from build123d import *

# Parameters (mm, degrees)
SKETCH1_W           = 85.2
SKETCH1_H           = 18
SKETCH1_R           = 1.5
BOSS_EXTRUDE1_DEPTH = 18
SKETCH2_R           = 3
CUT_EXTRUDE1_DEPTH  = 8
FILLET1_R           = 4


with BuildPart() as part:
    # Sketch1 → Boss-Extrude1 (new body)
    with BuildSketch(Plane(origin=(0, 0, 0), x_dir=(0, 0, -1), z_dir=(1, 0, 0))):
        with Locations((42.6, 9)):
            Rectangle(SKETCH1_W, SKETCH1_H)
        with Locations((76.2, 9)):
            Circle(SKETCH1_R, mode=Mode.SUBTRACT)
    extrude(amount=BOSS_EXTRUDE1_DEPTH)

    # Sketch2 → Cut-Extrude1 (cut)
    with BuildSketch(Plane.ZY):
        with Locations((-76.2, 9)):
            Circle(SKETCH2_R)
    extrude(amount=-CUT_EXTRUDE1_DEPTH, mode=Mode.SUBTRACT)

    # Fillet1
    fillet1_edges = [part.edges().sort_by_distance(p)[0] for p in [
        (9, 18, -85.2),
        (9, 0, -85.2),
    ]]
    fillet(fillet1_edges, radius=FILLET1_R)


solid = part.part
Input: part model. Units: mm. Frame: model coordinates. A direction names the side the tool comes from. Give positions to 0.01 mm unless a question says otherwise; leave off trailing zeros. Write each loop counter-clockwise with the first axis right and the second up, starting at its lowest first coordinate (ties: lowest second). Pieces come first, ordered by that corner, then holes.
Q1. Section A-A, the plane z = -76.2. Output: boundary loops of the cut face in (x, y), plus the area to 3 significant figures.
Q2. Set-up query: faces 5 (the face through (9.126, 16.859, -83.997)), 6 (the face through (8, 8, -78)). Return all of +Z, -Z, +X, -X, +Y, -Y with unobstructed straight access to the full face (end or side cutting, diameter ignored); none if empty.
Q3. Pull-direction query (Y, two-part tool) for faces 1 (the face through (3.94, 9.9, -73.34)), 2 (the face through (12.93, 7.67, -76.89)), 3 (the face through (18, 9, -42)), 4 (the face through (9, 0, -40)); classes: pulls with the +Y half, pulls with the -Y half, needs draft (parallel to the pull), parting line crosses it, or undercut.
Q4. Material intervals for probe 1 along Y at (x, z) = (15.25, -76.2); probe 2 along Y at (x, z) = (3.25, -76.2); probe 3 along Z at (x, y) = (13.5, 9), sorted ascending.
Q5. Section B-B, the plane y = 9. Output: boundary loops of the cut face in (x, z), plus the area to 3 significant figures.
Q6. First-contact query: P1, Ø2.5, axis at y = 9, z = -76.2, coming from the -X side. Flat tip, straight axial feed; report the tip coordinate or a pass-through.
Filled in:
1. outline: (0, 0) - (18, 0) - (18, 7.5) - (8, 7.5) - (8, 6) - (0, 6) - close; (0, 12) - (8, 12) - (8, 10.5) - (18, 10.5) - (18, 18) - (0, 18) - close
1. area: 246 mm2
2. face 5: -Z, +X, -X, +Y
2. face 6: -X
3. face 1: undercut
3. face 2: undercut
3. face 3: needs draft
3. face 4: pulls with the -Y half
4. probe 1: y = 0 to 7.5, 10.5 to 18
4. probe 2: y = 0 to 6, 12 to 18
4. probe 3: z = -85.2 to -77.7, -74.7 to 0
5. outline: (0, -85.2) - (18, -85.2) - (18, -77.7) - (8, -77.7) - (8, -79.2) - (0, -79.2) - close; (0, -73.2) - (8, -73.2) - (8, -74.7) - (18, -74.7) - (18, 0) - (0, 0) - close
5. area: 1,460 mm2
6. P1: passes through
